from build123d import *

# Parameters (mm, degrees)
CHAMFER1_SIZE       = 1
CUT_EXTRUDE6_DEPTH  = 130
CIRPATTERN1_COUNT   = 8
CUT_EXTRUDE8_DEPTH  = 10
SKETCH4_R           = 1.5
CUT_EXTRUDE9_DEPTH  = 15
SKETCH5_R           = 2.5
CUT_EXTRUDE10_DEPTH = 20
CUT_EXTRUDE11_DEPTH = 20


with BuildPart() as part:
    # Sketch1 → Revolve8 (revolve)
    with BuildSketch(Plane.XY):
        Polygon((0, 0), (10, 0), (10, 50), (25, 50), (25, 130), (12.5, 130), (12.5, 135), (10, 135), (10, 145), (12.5, 145), (12.5, 160), (0, 160), align=None)
    revolve(axis=Axis((0, 0, 0), (0, 1, 0)))

    # Chamfer1
    chamfer1_edges = [part.edges().sort_by_distance(p)[0] for p in [
        (-10, 0, 0),
    ]]
    chamfer(chamfer1_edges, length=CHAMFER1_SIZE)

    # Sketch2 → Cut-Extrude6 (cut)
    with BuildSketch(Plane(origin=(0, 0, 0), x_dir=(1, 0, 0), z_dir=(0, 1, 0))):
        with BuildLine():
            Line((24.874685928, 2.5), (20, 2.5))
            Line((20, 2.5), (20, 5))
            Line((20, 5), (15, 5))
            Line((15, 5), (15, -5))
            Line((15, -5), (20, -5))
            Line((20, -5), (20, -2.5))
            Line((20, -2.5), (24.874685928, -2.5))
            ThreePointArc((24.874685928, -2.5), (25, 0), (24.874685928, 2.5))
        make_face()
    cut_extrude6 = extrude(amount=CUT_EXTRUDE6_DEPTH, mode=Mode.SUBTRACT)

    # CirPattern1: Cut-Extrude6 ×8 about axis
    cirpattern1_axis = Axis((0, 0, 0), (0, 1, 0))
    for i in range(1, CIRPATTERN1_COUNT):
        add(cut_extrude6.rotate(cirpattern1_axis, i * 360 / CIRPATTERN1_COUNT), mode=Mode.SUBTRACT)

    # Sketch3 → Cut-Extrude8 (cut)
    with BuildSketch(Plane(origin=(0, 160, 0), x_dir=(1, 0, 0), z_dir=(0, 1, 0))):
        with BuildLine():
            Line((-7.5, 10), (7.5, 10))
            ThreePointArc((7.5, 10), (0, 12.5), (-7.5, 10))
        make_face()
        with BuildLine():
            Line((-10, 7.5), (-10, -7.5))
            ThreePointArc((-10, -7.5), (-12.5, 0), (-10, 7.5))
        make_face()
        with BuildLine():
            Line((-7.5, -10), (7.5, -10))
            ThreePointArc((7.5, -10), (0, -12.5), (-7.5, -10))
        make_face()
        with BuildLine():
            Line((10, 7.5), (10, -7.5))
            ThreePointArc((10, -7.5), (12.5, 0), (10, 7.5))
        make_face()
    extrude(amount=-CUT_EXTRUDE8_DEPTH, mode=Mode.SUBTRACT)

    # Sketch4 → Cut-Extrude9 (cut)
    with BuildSketch(Plane(origin=(0, 160, 0), x_dir=(1, 0, 0), z_dir=(0, 1, 0))):
        with Locations((-6, 6)):
            Circle(SKETCH4_R)
        with Locations((6, 6)):
            Circle(SKETCH4_R)
        with Locations((6, -6)):
            Circle(SKETCH4_R)
        with Locations((-6, -6)):
            Circle(SKETCH4_R)
    extrude(amount=-CUT_EXTRUDE9_DEPTH, mode=Mode.SUBTRACT)

    # Sketch5 → Cut-Extrude10 (cut)
    with BuildSketch(Plane.ZY.offset(10)):
        with Locations((0, 140)):
            Circle(SKETCH5_R)
    extrude(amount=-CUT_EXTRUDE10_DEPTH, mode=Mode.SUBTRACT)

    # Sketch6 → Cut-Extrude11 (cut)
    with BuildSketch(Plane.ZY.offset(10)):
        with BuildLine():
            Line((2.5, 32.5), (2.5, 7.5))
            ThreePointArc((2.5, 7.5), (0, 5), (-2.5, 7.5))
            Line((-2.5, 7.5), (-2.5, 32.5))
            ThreePointArc((-2.5, 32.5), (0, 35), (2.5, 32.5))
        make_face()
    extrude(amount=-CUT_EXTRUDE11_DEPTH, mode=Mode.SUBTRACT)


solid = part.part
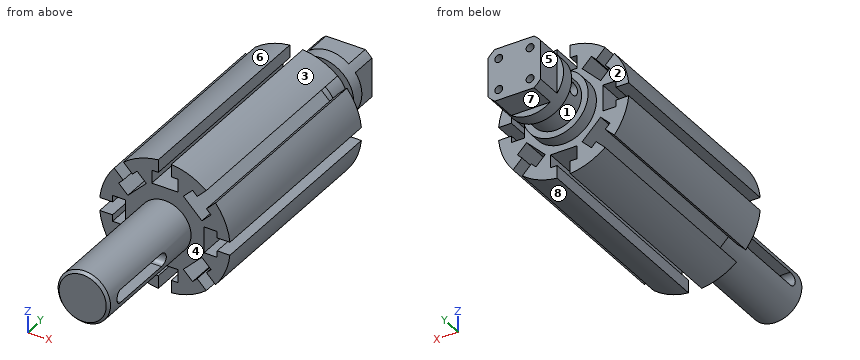
The model under review builds one solid part; all positions refer to its coordinate system, in mm. Face numbers are marked on the shaded views. A direction names the side the tool comes from. Give positions to 0.01 mm unless a question says otherwise; leave off trailing zeros. Loops run counter-clockwise (first coordinate to the right, second up) from the corner with the lowest first, then second, coordinate; pieces in that order, holes last. Notation, with made-up numbers: (89.25, 31.5) -> (112.25, 31.5) arc R18 ccw to (112.25, 44.5) -> close; hole circle Ø1 at (29.5, 21.5). An arc over 180 degrees is marked (long way). Answer as a JSON object with one key per item and string values. Group by question number.
Q1. Wall thickness on line 1 along X through (y, z) = (151.5, 6); line 2 along Y through (x, z) = (3, 0): over which ranges is each line inside the solid? List them lowest first.
Q2. Tool access review of the marked faces 4, 5, 6, 7 and 8: name each direction out of +Z, -Z, +X, -X, +Y, -Y from which nothing blocks a thin tool from reaching the whole face with its end or side.
Q3. Insertion check: pin 1 (2 mm diameter, centred on x = -3.5, y = 94.5, fed in from +Z); pin 2 (2.5 mm diameter, centred on x = 6, z = -6, fed in from +Y); pin 3 (1.5 mm diameter, centred on y = 93.5, z = 16.5, fed in from +X); pin 4 (1.5 mm diameter, centred on y = 100.5, z = -22.5, fed in from +X). Each pin has a flat end and moves straight along its axis. Give the tip position at first contact, or say it passes through.
Q4. Take a section at B-B (x = -22). Write out the cut boundary in (y, z).
Q5. Take a section at A-A (x = 0). State how many separate pieces and enclosed holes the cut face has, plus the area to 3 significant figures.
Q6. Draft analysis for pull direction Y (two halves, no side actions). For the marked faces 1, 2 and 3, state which applies: pulls with the +Y half, pulls with the -Y half, needs draft (parallel to the pull), parting line crosses it, or undercut.
Q7. Take a section at C-C (y = 140). Write out the cut boundary in (x, z).
Answer below:
{
 "1": {"line 1": "x = -10 to -7.5, -4.5 to 4.5, 7.5 to 10", "line 2": "y = 0 to 5, 35 to 137.5, 142.5 to 160"},
 "2": {"face 4": "-Y", "face 5": "+Z, -Z, -X, +Y", "face 6": "+Z, -X, +Y, -Y", "face 7": "-Z, +X, -X, +Y", "face 8": "-Z, +X, +Y, -Y"},
 "3": {"pin 1": "stops at z = 24.87", "pin 2": "stops at y = 145", "pin 3": "stops at x = 19.41", "pin 4": "stops at x = 12.33"},
 "4": {"outline": "(50, -11.87) -> (130, -11.87) -> (130, -2.5) -> (50, -2.5) -> close; (50, 2.5) -> (130, 2.5) -> (130, 11.87) -> (50, 11.87) -> close"},
 "5": {"separate pieces": "1", "enclosed holes": "2", "area": "3,880 mm2"},
 "6": {"face 1": "undercut", "face 2": "pulls with the +Y half", "face 3": "needs draft"},
 "7": {"outline": "(-9.68, -2.5) arc R10 ccw to (9.68, -2.5) -> close; (-9.68, 2.5) -> (9.68, 2.5) arc R10 ccw to start"}
}
